Input: dimensioned drawing with shaded views. Units: mm. Origin: part minimum x, y, z. A direction names the side the tool comes from. Coordinates: 2 decimals unless noted, no trailing zeros. Order: outer loops, then holes, each group sorted by start corner. A loop starts at its lowest first (then second) coordinate and runs counter-clockwise, first axis right, second up. Notation, with made-up numbers: (39.25, -39.5) - (61.25, -39.5) arc R29 cw to (61.25, -7.5) - close; hole circle Ø3 at (-0.75, -34). An arc over 180 degrees is marked (long way). One line per question, with ' | ' between items. Start each with the question number.
(1) Section B-B (y = 28.7). Return the cut outline in (x, z), then the cut area to 3 significant figures.
(2) Contact query for flat-ended pins moving along their axis: P1, Ø8, axis at y = 45, z = 38.5, coming from the -X side; P2, Ø1, axis at y = 15, z = 46, coming from the -X side; P3, Ø6, axis at x = 5.2, y = 52.2, coming from the +Z side. Output: stop coordinate, or through.
(3) Line query: line 1 along Y through (x, z) = (5.2, 3.5); line 2 along X through (y, z) = (5, 52); line 3 along Z through (x, y) = (7.5, 50). Output: solid intervals per line, ascending.
(4) Section D-D (z = 69). Return the cut outline in (x, y).
(5) Section C-C (x = 19.5). Return the cut outline in (y, z).
(6) Draft query along Z for the marked faces 1, 2 and 3. Return one class per face: +Z half, -Z half, draft (parallel to the pull), parting line (faces both ways), or undercut.
(7) Access query for the marked faces 4 and 5. Directions: +Z, -Z, +X, -X, +Y, -Y. A direction counts if a zero-diameter tool reaches every point of the face in a straight line with its end or side. Return the directions, or none.
(8) Section A-A (y = 53.5). Return the cut outline in (x, z), then the cut area to 3 significant figures.
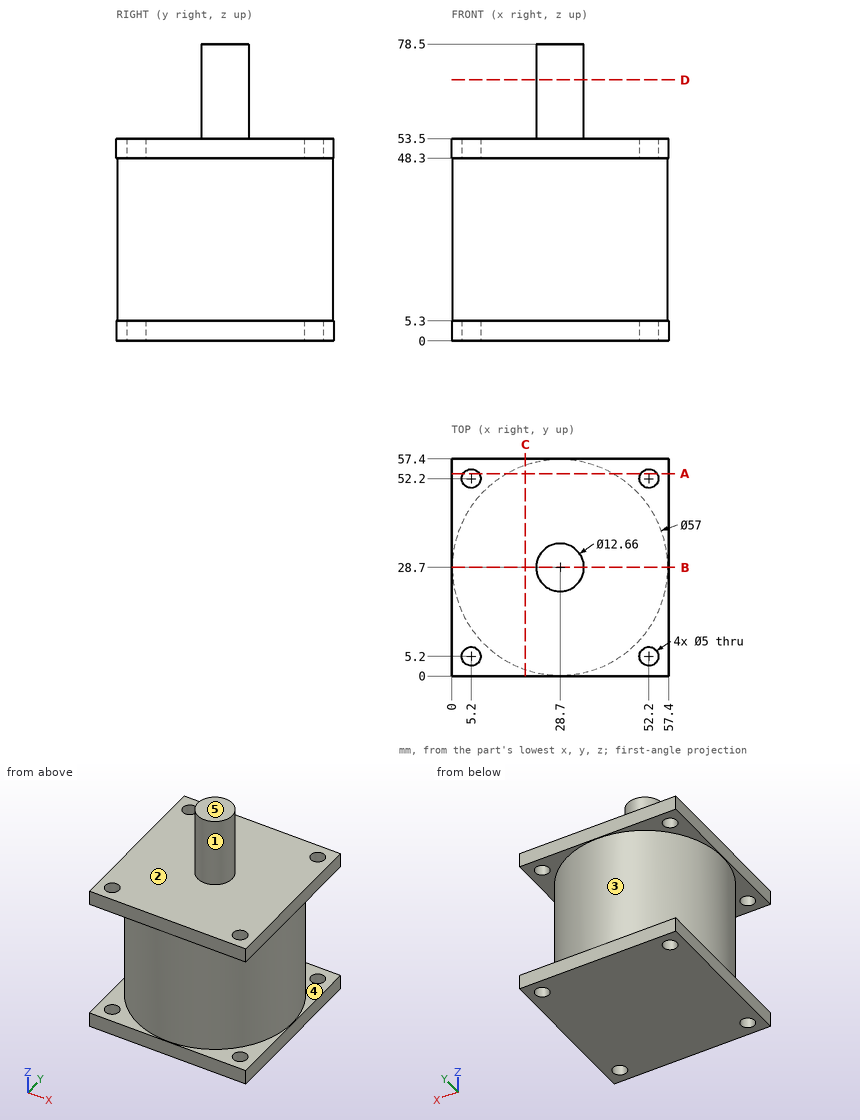
Response values:
1) outline: (0, 0) - (57.4, 0) - (57.4, 5.3) - (57.2, 5.3) - (57.2, 48.3) - (57.4, 48.3) - (57.4, 53.5) - (35.03, 53.5) - (35.03, 78.5) - (22.37, 78.5) - (22.37, 53.5) - (0, 53.5) - (0, 48.3) - (0.2, 48.3) - (0.2, 5.3) - (0, 5.3) - close | area: 3,370 mm²
2) P1: stops at x = 2.99 | P2: stops at x = 3.44 | P3: stops at z = 53.5
3) line 1: y = 0 to 2.7, 7.7 to 49.7, 54.7 to 57.4 | line 2: x = 0 to 2.71, 7.69 to 49.71, 54.69 to 57.4 | line 3: z = 0 to 5.3, 48.3 to 53.5
4) outline: circle Ø12.66 at (28.7, 28.7)
5) outline: (0, 0) - (57.4, 0) - (57.4, 5.3) - (55.67, 5.3) - (55.67, 48.3) - (57.4, 48.3) - (57.4, 53.5) - (0, 53.5) - (0, 48.3) - (1.73, 48.3) - (1.73, 5.3) - (0, 5.3) - close
6) face 1: draft | face 2: +Z half | face 3: undercut
7) face 4: none | face 5: +Z, +X, -X, +Y, -Y
8) outline: (0, 0) - (3.06, 0) - (3.06, 5.3) - (0, 5.3) - close; (0, 48.3) - (3.06, 48.3) - (3.06, 53.5) - (0, 53.5) - close; (7.34, 0) - (50.06, 0) - (50.06, 5.3) - (42.74, 5.3) - (42.74, 48.3) - (50.06, 48.3) - (50.06, 53.5) - (7.34, 53.5) - (7.34, 48.3) - (14.66, 48.3) - (14.66, 5.3) - (7.34, 5.3) - close; (54.34, 0) - (57.4, 0) - (57.4, 5.3) - (54.34, 5.3) - close; (54.34, 48.3) - (57.4, 48.3) - (57.4, 53.5) - (54.34, 53.5) - close | area: 1,720 mm²
